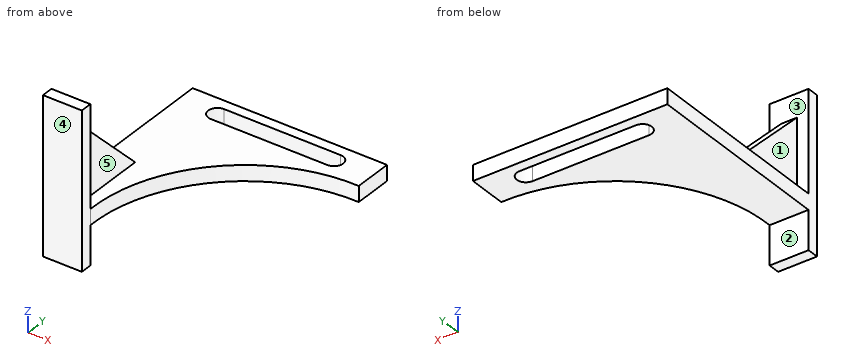
from build123d import *

# Parameters (mm, degrees)
SKETCH1_W           = 50
SKETCH1_H           = 200
BOSS_EXTRUDE1_DEPTH = 15
BOSS_EXTRUDE2_DEPTH = 20
BOSS_EXTRUDE3_DEPTH = 10
CUT_EXTRUDE1_DEPTH  = 71


with BuildPart() as part:
    # Sketch1 → Boss-Extrude1 (new body)
    with BuildSketch(Plane(origin=(0, 0, 0), x_dir=(1, 0, 0), z_dir=(0, 1, 0))):
        Rectangle(SKETCH1_W, SKETCH1_H)
    extrude(amount=BOSS_EXTRUDE1_DEPTH)

    # Sketch2 → Boss-Extrude2 (add)
    with BuildSketch(Plane.XY.offset(-50)):
        with BuildLine():
            Line((-25, 15), (-25, 265))
            Line((-25, 265), (225, 265))
            Line((225, 265), (225, 215))
            ThreePointArc((225, 215), (82.144079422, 157.855920578), (25, 15))
            Line((25, 15), (-25, 15))
        make_face()
    extrude(amount=BOSS_EXTRUDE2_DEPTH)

    # Sketch3 → Boss-Extrude3 (add, symmetric)
    with BuildSketch(Plane(origin=(0, 0, 0), x_dir=(0, 0, -1), z_dir=(1, 0, 0))):
        Polygon((-70, 15), (30, 15), (30, 115), align=None)
    extrude(amount=BOSS_EXTRUDE3_DEPTH, both=True)

    # Sketch4 → Cut-Extrude1 (cut, through all)
    with BuildSketch(Plane.XY.offset(-30)):
        with BuildLine():
            Line((25, 228.25), (175, 228.25))
            ThreePointArc((175, 228.25), (186.75, 240), (175, 251.75))
            Line((175, 251.75), (25, 251.75))
            ThreePointArc((25, 251.75), (13.25, 240), (25, 228.25))
        make_face()
    extrude(amount=-CUT_EXTRUDE1_DEPTH, mode=Mode.SUBTRACT)


solid = part.part
Part model, mm, in its own coordinate system. Face numbers are marked on the shaded views. A direction names the side the tool comes from. Give positions to 0.01 mm unless a question says otherwise; leave off trailing zeros. Order: outer loops, then holes, each group sorted by start corner. A loop starts at its lowest first (then second) coordinate and runs counter-clockwise, first axis right, second up. Notation, with made-up numbers: (68.25, 34.25) -> (116.25, 34.25) arc R16 ccw to (116.25, 44.25) -> close; hole circle Ø10 at (76, 29.5). An arc over 180 degrees is marked (long way). Use one line per item in the form item = value.
(1) Drill centre lines: line 1 (Y direction, x = 10, z = -89.5); line 2 (X direction, y = 28, z = 20.5); line 3 (Z direction, x = 12.5, y = 62.5). Where is each one in solid material? Low to high. Write a range as from..to.
Solution:
line_1 = 0..15
line_2 = -10..10
line_3 = -50..-30
(2) Saw through at D-D (x = 124). Write the cut outline in (y, z).
Solution:
outline = (189.7, -50) -> (228.25, -50) -> (228.25, -30) -> (189.7, -30) -> close; (251.75, -50) -> (265, -50) -> (265, -30) -> (251.75, -30) -> close
(3) Saw through at B-B (z = -35). Write the cut outline in (x, y), then the cut area to 3 significant figures.
Solution:
outline = (-25, 0) -> (25, 0) -> (25, 15) arc R195.3 cw to (225, 215) -> (225, 265) -> (-25, 265) -> close; hole (25, 228.25) -> (175, 228.25) arc R11.75 ccw to (175, 251.75) -> (25, 251.75) arc R11.75 ccw to start
area = 27,500 mm²
(4) Saw through at C-C (x = -1). Write the cut outline in (y, z).
Solution:
outline = (0, -100) -> (15, -100) -> (15, -50) -> (265, -50) -> (265, -30) -> (115, -30) -> (15, 70) -> (15, 100) -> (0, 100) -> close
(5) Flat gauge pins, fed straight in: P1, Ø6, axis at x = 5, z = 53.5, coming from the +Y side; P2, Ø1, axis at x = 34.5, y = 106, coming from the +Z side; P3, Ø10, axis at x = 115, z = -38, coming from the -Y side. Where does each tip first touch, or does it go through?
Solution:
P1 = 34.5
P2 = -30
P3 = 180.97
(6) Tool access for the marked faces 1, 2, 3, 4 and 5: list every direction of +Z, -Z, +X, -X, +Y, -Y with a clear straight run to the whole face (end or side of a thin tool).
Solution:
face_1 = +Z, -X, +Y
face_2 = -Z, +X, -X, +Y
face_3 = +Z, +Y
face_4 = +Z, -Z, +X, -X, -Y
face_5 = +Z, +X, +Y
(7) Saw through at A-A (y = 240). Write the cut outline in (x, z).
Solution:
outline = (-25, -50) -> (13.25, -50) -> (13.25, -30) -> (-25, -30) -> close; (186.75, -50) -> (225, -50) -> (225, -30) -> (186.75, -30) -> close
